```python
from build123d import *

# Parameters (mm, degrees)
F0_R      = 5
F1_DEPTH  = 4
F3_R      = 1
F4_R      = 1.5
F5_DEPTH  = 1.5
F6_R      = 1.48
F7_R      = 1
F8_R      = 1
F9_DEPTH  = 4
F10_DEPTH = 4
F12_DEPTH = 25
F13_DEPTH = 25
F14_DEPTH = 25
F15_DEPTH = 25
F16_DEPTH = 25
F17_DEPTH = 25
F18_DEPTH = 25
F19_DEPTH = 25
F20_DEPTH = 25
F21_DEPTH = 25
F22_SIZE2 = 3.3107096722
F22_SIZE  = 2.15
F23_SIZE2 = 2.3975903424
F23_SIZE  = 3.3
F24_SIZE2 = 10.1563556727
F24_SIZE  = 3.3


with BuildPart() as f1:
    # F0 (on Front) → F1 (new body)
    with BuildSketch(Plane.XZ):
        Polygon((-5.0394813192, 34.4464560161), (-11.4673425455, 30.2002090896), (-11.4673425455, 14.3180689151), (-9.5205468137, 12.9544524784), (-9.5205468137, 5.9659214999), (-11.4673425455, 4.6023059945), (-11.4673425455, -3.5793893662), (-9.5205468137, -4.943005803), (-9.5205468137, -11.4201806177), (-11.4673425455, -12.7837961231), (-11.4673425455, -24.7997909104), (-3.8956315734, -25.2267909859), (0.1954483631, -11.7619743544), (-3.008507374, -6.1141202787), (-5.1672247355, -2.308786607), (-2.9510677868, 1.4633843035), (1.4238065236, 1.4302215424), (3.2341110933, -1.7609386613), (5.9812411675, 7.2805866294), (4.9106002387, 10.2737202031), (5.3487122304, 11.715661628), (6.5019388672, 15.5112328316), (8.8668211656, 16.7777869175), (13.660922366, 32.55643084), (7.090733743, 35.8415256189), (1.388379907, 38.6927029426), align=None)
        with Locations((-2.1907666232, 11.0733276233)):
            Circle(F0_R, mode=Mode.SUBTRACT)
    extrude(amount=F1_DEPTH)

    # F3
    f3_edges = [f1.edges().sort_by_distance(p)[0] for p in [
        (-11.467343, -2, 30.200209),
        (13.660922, -2, 32.556431),
    ]]
    fillet(f3_edges, radius=F3_R)

    # F4
    f4_edges = [f1.edges().sort_by_distance(p)[0] for p in [
        (1.38838, -2, 38.692703),
    ]]
    fillet(f4_edges, radius=F4_R)

    # F0 (on Front) → F5 (join)
    with BuildSketch(Plane.XZ):
        Polygon((-5.0394813192, 36.4464560161), (-5.0394813192, 34.4464560161), (1.388379907, 38.6927029426), (7.090733743, 35.8415256189), (7.090733743, 37.8415256189), (1.3569573109, 40.6719451668), align=None)
    extrude(amount=F5_DEPTH)

    # F6
    f6_edges = [f1.edges().sort_by_distance(p)[0] for p in [
        (1.38838, -0.75, 38.692703),
    ]]
    fillet(f6_edges, radius=F6_R)

    # F7
    f7_edges = [f1.edges().sort_by_distance(p)[0] for p in [
        (1.356957, -0.75, 40.671945),
    ]]
    fillet(f7_edges, radius=F7_R)

    # F8
    f8_edges = [f1.edges().sort_by_distance(p)[0] for p in [
        (7.090734, -0.75, 37.841526),
        (-5.039481, -0.75, 36.446456),
    ]]
    fillet(f8_edges, radius=F8_R)

    # F0 (on Front) → F9 (join)
    with BuildSketch(Plane.XZ):
        Polygon((-9.5205468137, 12.9544524784), (-11.4673425455, 14.3180689151), (-11.4673425455, 4.6023059945), (-9.5205468137, 5.9659214999), align=None)
    extrude(amount=F9_DEPTH)

    # F0 (on Front) → F10 (join)
    with BuildSketch(Plane.XZ):
        Polygon((-9.5205468137, -4.943005803), (-11.4673425455, -3.5793893662), (-11.4673425455, -12.7837961231), (-9.5205468137, -11.4201806177), align=None)
    extrude(amount=F10_DEPTH)

    # F11 (on face) → F12 (cut)
    with BuildSketch(Plane.XZ.offset(4)):
        Polygon((-11.4673425455, 18.1700624526), (-11.4673425455, 8.4008118138), (-9.4790116895, 9.7482940182), (-9.4790116895, 16.8225802481), align=None)
    extrude(amount=-F12_DEPTH, mode=Mode.SUBTRACT)

    # F11 (on face) → F13 (cut)
    with BuildSketch(Plane.XZ.offset(4)):
        Polygon((-11.4673425455, 2.4312612155), (-11.4673425455, -7.9374192283), (-9.3105754826, -6.4215008169), (-9.3105754826, 0), align=None)
    extrude(amount=-F13_DEPTH, mode=Mode.SUBTRACT)

    # F2 (on face) → F14 (cut)
    with BuildSketch(Plane.XZ.offset(4)):
        Polygon((4.8250659445, 23.1876130557), (6.5640832201, 28.4046710308), (3.0962773256, 32.3153540431), (-1.2611432737, 31.4323578126), (-1.8441430637, 29.694451147), (0.58299979, 26.9467592245), (-0.58299979, 23.4709458933), (0.456882035, 22.2937284557), align=None)
    extrude(amount=-F14_DEPTH, mode=Mode.SUBTRACT)

    # F2 (on face) → F15 (cut)
    with BuildSketch(Plane.XZ.offset(4)):
        Polygon((-4.3431362726, 22.9318731841), (-1.7787461332, 23.4566379151), (-4.2111435343, 26.1996793323), (-3.1332999575, 29.4332138733), (-5.4372854972, 28.9663297384), (-6.6032850771, 25.4905164073), align=None)
    extrude(amount=-F15_DEPTH, mode=Mode.SUBTRACT)

    # F2 (on face) → F16 (cut)
    with BuildSketch(Plane.XZ.offset(4)):
        Polygon((-3.0101426436, 26.2186378159), (-1.4476834802, 24.4498270447), (-0.6194012828, 26.9346765651), (-2.1796810883, 28.6942213364), align=None)
    extrude(amount=-F16_DEPTH, mode=Mode.SUBTRACT)

    # F2 (on face) → F17 (cut)
    with BuildSketch(Plane.XZ.offset(4)):
        Polygon((-1.7787461332, 23.4566379151), (-1.4476834802, 24.4498270447), (-3.0101426436, 26.2186378159), (-2.1796810883, 28.6942213364), (-2.8804242206, 29.4844571071), (-3.1332999575, 29.4332138733), (-4.2111435343, 26.1996793323), align=None)
    extrude(amount=-F17_DEPTH, mode=Mode.SUBTRACT)

    # F2 (on face) → F18 (cut)
    with BuildSketch(Plane.XZ.offset(4)):
        Polygon((-1.4476834802, 24.4498270447), (-0.58299979, 23.4709458933), (0.58299979, 26.9467592245), (-1.8441430637, 29.694451147), (-2.1796810883, 28.6942213364), (-0.6194012828, 26.9346765651), align=None)
    extrude(amount=-F18_DEPTH, mode=Mode.SUBTRACT)

    # F2 (on face) → F19 (cut)
    with BuildSketch(Plane.XZ.offset(4)):
        Polygon((-2.1796810883, 28.6942213364), (-1.8441430637, 29.694451147), (-2.8804242206, 29.4844571071), align=None)
    extrude(amount=-F19_DEPTH, mode=Mode.SUBTRACT)

    # F2 (on face) → F20 (cut)
    with BuildSketch(Plane.XZ.offset(4)):
        Polygon((-1.6073627495, 23.2633669802), (-0.58299979, 23.4709458933), (-1.4476834802, 24.4498270447), (-1.7787461332, 23.4566379151), align=None)
    extrude(amount=-F20_DEPTH, mode=Mode.SUBTRACT)

    # F2 (on face) → F21 (cut)
    with BuildSketch(Plane.XZ.offset(4)):
        Polygon((-4.1761422235, 22.7428244847), (-1.6073627495, 23.2633669802), (-1.7787461332, 23.4566379151), (-4.3431362726, 22.9318731841), align=None)
    extrude(amount=-F21_DEPTH, mode=Mode.SUBTRACT)

    # F22
    f22_edges = [f1.edges().sort_by_distance(p)[0] for p in [
        (-11.467343, -4, -16.368605),
    ]]
    chamfer(f22_edges, length=F22_SIZE, length2=F22_SIZE2)

    # F23
    f23_edges = [f1.edges().sort_by_distance(p)[0] for p in [
        (-1.850092, -4, -18.494383),
    ]]
    f23_side = f1.faces().sort_by_distance((-1.850092, -2, -18.494383))[0]
    chamfer(f23_edges, length=F23_SIZE, length2=F23_SIZE2, reference=f23_side)

    # F24
    f24_edges = [f1.edges().sort_by_distance(p)[0] for p in [
        (-7.838288, -4, -25.004448),
    ]]
    f24_side = f1.faces().sort_by_distance((-7.731254, -1.697794, -25.010484))[0]
    chamfer(f24_edges, length=F24_SIZE, length2=F24_SIZE2, reference=f24_side)


solid = f1.part
```
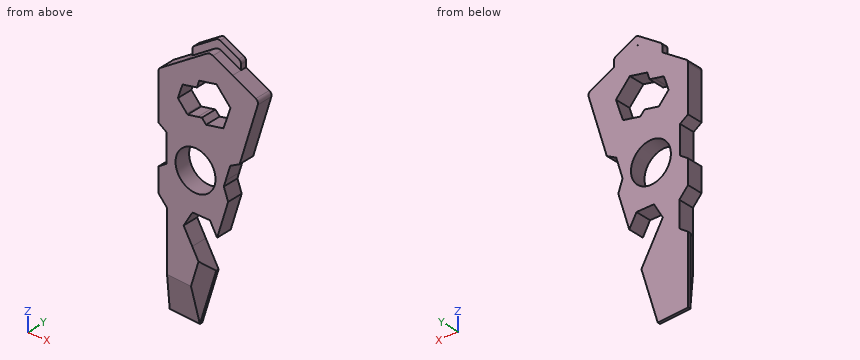
Read the model definition and answer for the solid it produces. Units are mm, in the model's axes. Give positions to 0.01 mm unless a question says otherwise; leave off trailing zeros. Order: outer loops, then holes, each group sorted by start corner. A loop starts at its lowest first (then second) coordinate and runs counter-clockwise, first axis right, second up. Notation, with made-up numbers: (53, -18.75) -> (106, -18.75) arc R13 cw to (106, -14.75) -> close; hole circle Ø3 at (-39.75, 85.25). An arc over 180 degrees is marked (long way). Write item = value, one per line.
1. A cutting plane is placed at B-B, the plane x = -8.5. Write down the section's boundary in (y, z).
Numbers:
outline = (-4, -14.79) -> (-0.7, -24.97) -> (0, -24.97) -> (0, 32.16) -> (-4, 32.16) -> close
2. Given pin 1 (1.2 mm diameter, centred on y = -2, z = -4.5, fed in from -X); pin 2 (0.7 mm diameter, centred on y = -1, z = 35, fed in from -X); pin 3 (1 mm diameter, centred on x = -5, y = -0.5, fed in from -Z), each flat-ended and moving along its own axis, determine where each tip first touches the part or whether it passes through.
Numbers:
pin_1 = -9.31
pin_2 = -5.04
pin_3 = -25.19
3. A cutting plane is placed at D-D, the plane x = 11.25. Write down the section's boundary in (y, z).
Numbers:
outline = (-4, 24.62) -> (0, 24.62) -> (0, 33.76) -> (-4, 33.76) -> close
4. A cutting plane is placed at C-C, the plane y = -2.45. Count the separate pieces of the cut face and the enclosed holes in it, and give its area (3 significant figures).
Numbers:
separate_pieces = 1
enclosed_holes = 2
area = 653 mm²
5. Straight lines are drawn through the part: line 1 along Z through (x, y) = (-0.75, -3.6); line 2 along X through (y, z) = (-1.9, 24); line 3 along X through (y, z) = (-1.15, 8). For each, find the intervals that lie inside material, in ascending order.
Numbers:
line_1 = 1.45 to 6.29, 15.86 to 23.44, 31.54 to 37.28
line_2 = -11.47 to -5.29, 5.1 to 11.06
line_3 = -11.47 to -6.13, 1.75 to 5.72
6. A cutting plane is placed at A-A, the plane z = -16.5. Write down the section's boundary in (x, y), and give its area (3 significant figures).
Numbers:
outline = (-11.47, -0.69) -> (-9.69, -3.42) -> (-3.4, -3.54) -> (-1.24, -0.7) -> (-1.24, 0) -> (-11.47, 0) -> close
area = 30.1 mm²
